The listing builds one solid part. Answer for the finished solid, in the listing's coordinates (mm). Coordinates: 2 decimals unless noted, no trailing zeros. Loops run counter-clockwise (first coordinate to the right, second up) from the corner with the lowest first, then second, coordinate; pieces in that order, holes last. Notation, with made-up numbers: (61, 8) - (79, 8) arc R24 ccw to (79, 25) - close; hole circle Ø10 at (72, 80). An arc over 180 degrees is marked (long way). Write each question's results on one line, items separated by ' | '. Start each with the question number.
(1) Find section C-C on x = 35.56. Determine the outline of the cut face in (y, z) (3 decimals), then the cut area to 3 significant figures.
(2) Given pin 1 Ø3 at (x, y) = (-17.78, 36.83) entering from +Z, flat-ended and moving along its own axis, determine where the tip first touches the part or whether it passes through.
(3) Find section D-D on z = 1.5. Determine the outline of the cut face in (x, y), then the cut area to 3 significant figures.
(4) Find section A-A on y = 36.83. Determine the outline of the cut face in (x, z) (3 decimals), then the cut area to 3 significant figures.
(5) Consider line 1 (Y direction, x = -7.5, z = 0.25); line 2 (Y direction, x = -17.78, z = 1.15); line 3 (X direction, y = -62, z = 2.55). Determine where each line is inside the solid, lowest interval first. Write a range as from..to.
(6) Find section B-B on x = -13. Determine the outline of the cut face in (y, z) (3 decimals).
from build123d import *

# Parameters (mm, degrees)
F0_W     = 203.2
F0_H     = 152.4
F0_W_2   = 177.8
F0_H_2   = 12.7
F0_R     = 2.54
F1_DEPTH = 3.175


# Not quite as in the source:
# - a length typed as a fraction of an inch, garbled in the dataset ("3 / 203.2 mm" for 3/8 in), is restored
# - a feature names something its author has since deleted; it is built from what else it names


with BuildPart() as f1:
    # F0 (on Top) → F1 (new body)
    with BuildSketch(Plane.XY):
        Rectangle(F0_W, F0_H)
        with Locations((0, -57.15)):
            Rectangle(F0_W_2, F0_H_2, mode=Mode.SUBTRACT)
        with Locations((-17.78, -36.83)):
            Circle(F0_R, mode=Mode.SUBTRACT)
        with Locations((35.56, -36.83)):
            Circle(F0_R, mode=Mode.SUBTRACT)
        with Locations((-17.78, 36.83)):
            Circle(F0_R, mode=Mode.SUBTRACT)
        with Locations((0, 57.15)):
            Rectangle(F0_W_2, F0_H_2, mode=Mode.SUBTRACT)
        with Locations((35.56, 36.83)):
            Circle(F0_R, mode=Mode.SUBTRACT)
    extrude(amount=F1_DEPTH)


solid = f1.part
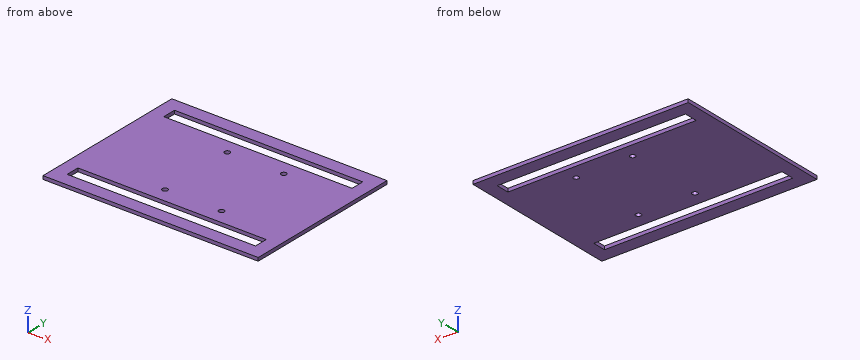
Values:
1) outline: (-76.2, 0) - (-63.5, 0) - (-63.5, 3.175) - (-76.2, 3.175) - close; (-50.8, 0) - (-39.37, 0) - (-39.37, 3.175) - (-50.8, 3.175) - close; (-34.29, 0) - (34.29, 0) - (34.29, 3.175) - (-34.29, 3.175) - close; (39.37, 0) - (50.8, 0) - (50.8, 3.175) - (39.37, 3.175) - close; (63.5, 0) - (76.2, 0) - (76.2, 3.175) - (63.5, 3.175) - close | area: 371 mm²
2) pin 1: passes through
3) outline: (-101.6, -76.2) - (101.6, -76.2) - (101.6, 76.2) - (-101.6, 76.2) - close; hole (-88.9, -63.5) - (88.9, -63.5) - (88.9, -50.8) - (-88.9, -50.8) - close; hole (-88.9, 50.8) - (88.9, 50.8) - (88.9, 63.5) - (-88.9, 63.5) - close; hole circle Ø5.08 at (-17.78, -36.83); hole circle Ø5.08 at (-17.78, 36.83); hole circle Ø5.08 at (35.56, -36.83); hole circle Ø5.08 at (35.56, 36.83) | area: 26,400 mm²
4) outline: (-101.6, 0) - (-20.32, 0) - (-20.32, 3.175) - (-101.6, 3.175) - close; (-15.24, 0) - (33.02, 0) - (33.02, 3.175) - (-15.24, 3.175) - close; (38.1, 0) - (101.6, 0) - (101.6, 3.175) - (38.1, 3.175) - close | area: 613 mm²
5) line 1: y = -76.2..-63.5, -50.8..50.8, 63.5..76.2 | line 2: y = -76.2..-63.5, -50.8..-39.37, -34.29..34.29, 39.37..50.8, 63.5..76.2 | line 3: x = -101.6..-88.9, 88.9..101.6
6) outline: (-76.2, 0) - (-63.5, 0) - (-63.5, 3.175) - (-76.2, 3.175) - close; (-50.8, 0) - (50.8, 0) - (50.8, 3.175) - (-50.8, 3.175) - close; (63.5, 0) - (76.2, 0) - (76.2, 3.175) - (63.5, 3.175) - close
